```python
from build123d import *

# Parameters (mm, degrees)
SKETCH1_W           = 90
SKETCH1_H           = 20
BOSS_EXTRUDE1_DEPTH = 1
SKETCH2_R           = 2
CUT_EXTRUDE1_DEPTH  = 2
FILLET1_R           = 3
SKETCH3_W           = 74
SKETCH3_H           = 5.275339083
BOSS_EXTRUDE2_DEPTH = 8
SKETCH4_W           = 16
SKETCH4_H           = 3
BOSS_EXTRUDE3_DEPTH = 4
SKETCH5_W           = 4
SKETCH5_H           = 1.5
BOSS_EXTRUDE4_DEPTH = 10
SKETCH6_W           = 24
SKETCH6_H           = 11
BOSS_EXTRUDE5_DEPTH = 10
CUT_EXTRUDE2_DEPTH  = 12


with BuildPart() as part:
    # Sketch1 → Boss-Extrude1 (new body)
    with BuildSketch(Plane(origin=(0, 0, 0), x_dir=(1, 0, 0), z_dir=(0, 1, 0))):
        with Locations((45, 10)):
            Rectangle(SKETCH1_W, SKETCH1_H)
    extrude(amount=BOSS_EXTRUDE1_DEPTH)

    # Sketch2 → Cut-Extrude1 (cut, through all)
    with BuildSketch(Plane(origin=(0, 1, 0), x_dir=(1, 0, 0), z_dir=(0, 1, 0))):
        with Locations((3, 17)):
            Circle(SKETCH2_R)
        with Locations((87, 17)):
            Circle(SKETCH2_R)
        with Locations((87, 3)):
            Circle(SKETCH2_R)
        with Locations((3, 3)):
            Circle(SKETCH2_R)
    extrude(amount=-CUT_EXTRUDE1_DEPTH, mode=Mode.SUBTRACT)

    # Fillet1
    fillet1_edges = [part.edges().sort_by_distance(p)[0] for p in [
        (0, 0.5, -20),
        (90, 0.5, -20),
        (90, 0.5, 0),
        (0, 0.5, 0),
    ]]
    fillet(fillet1_edges, radius=FILLET1_R)

    # Sketch3 → Boss-Extrude2 (add)
    with BuildSketch(Plane(origin=(0, 1, 0), x_dir=(1, 0, 0), z_dir=(0, 1, 0))):
        with Locations((45, 15.362330459)):
            Rectangle(SKETCH3_W, SKETCH3_H)
    extrude(amount=BOSS_EXTRUDE2_DEPTH)

    # Sketch4 → Boss-Extrude3 (add)
    with BuildSketch(Plane(origin=(0, 1, 0), x_dir=(1, 0, 0), z_dir=(0, 1, 0))):
        with Locations((16, 2.5)):
            Rectangle(SKETCH4_W, SKETCH4_H)
    extrude(amount=BOSS_EXTRUDE3_DEPTH)

    # Sketch5 → Boss-Extrude4 (add)
    with BuildSketch(Plane(origin=(0, 9, 0), x_dir=(1, 0, 0), z_dir=(0, 1, 0))):
        with Locations((25, 15.362330459)):
            Rectangle(SKETCH5_W, SKETCH5_H)
    extrude(amount=BOSS_EXTRUDE4_DEPTH)

    # Sketch6 → Boss-Extrude5 (add)
    with BuildSketch(Plane(origin=(0, 19, 0), x_dir=(1, 0, 0), z_dir=(0, 1, 0))):
        with Locations((25, 15.362330459)):
            Rectangle(SKETCH6_W, SKETCH6_H)
    extrude(amount=BOSS_EXTRUDE5_DEPTH)

    # Sketch7 → Cut-Extrude2 (cut, through all)
    with BuildSketch(Plane.XY.offset(-9.862330459)):
        Polygon((37, 29), (25, 25.5), (13, 29), align=None)
    extrude(amount=-CUT_EXTRUDE2_DEPTH, mode=Mode.SUBTRACT)


solid = part.part
```
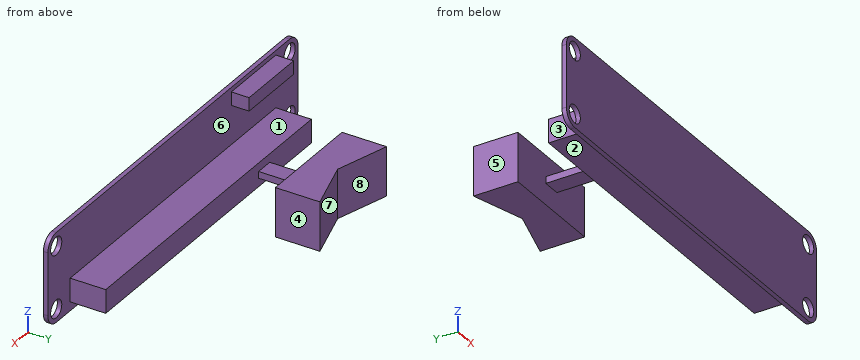
Part model, mm, in its own coordinate system. Face numbers are marked on the shaded views. A direction names the side the tool comes from. Round coordinates to 2 decimals unless told otherwise and drop trailing zeros. Order: outer loops, then holes, each group sorted by start corner. A loop starts at its lowest first (then second) coordinate and runs counter-clockwise, first axis right, second up. Notation, with made-up numbers: M 62.25,-1 L 101.25,-1 A21 cw 101.25,20 Z; hole C -29,30 d11. An arc over 180 degrees is marked long. Put each result on its own line as item: value. Start each with the question number.
1. Two-plate mould, pull along X, no slides. Class the marked faces 5, 6, 7 and 8: +X half, -X half, draft (parallel to the pull), parting line (faces both ways), or undercut.
2. Drop flat-ended pins along their axis: pin 1 (2 mm diameter, centred on x = 24, y = 12, fed in from +Z); pin 2 (1.6 mm diameter, centred on y = 12, z = -15, fed in from +X); pin 3 (4.5 mm diameter, centred on x = 19, y = 3, fed in from -Z). Give the stop position or say it passes through.
3. Tool access for the marked faces 1, 2, 3 and 4: list every direction of +Z, -Z, +X, -X, +Y, -Y with a clear straight run to the whole face (end or side of a thin tool).
4. Slice it at C-C on x = 29.5. List the corners of the cut face in (y, z).
5. Slice it at A-A on y = 2.75. List the corners of the cut face in (x, z).
6. Slice it at B-B on x = 18. List the corners of the cut face in (y, z).
7. Slice it at D-D on z = -6.25. List the corners of the cut face in (x, y).
8. Drill centre lines: probe 1 along Z at (x, y) = (87, 0.45); probe 2 along X at (y, z) = (0.85, -17); probe 3 along Y at (x, z) = (85, -12.5). Where is each one in solid material? Low to high. Write a range as [from, to].
Findings:
1. face 5: -X half
1. face 6: draft
1. face 7: undercut
1. face 8: undercut
2. pin 1: z = -14.61
2. pin 2: x = 27
2. pin 3: z = -20
3. face 1: +X, -X
3. face 2: -Z, +X, -X
3. face 3: +Z, -Z, -X, +Y
3. face 4: +Z, -Z, +X, +Y
4. outline: M 0,-20 L 1,-20 L 1,-18 L 9,-18 L 9,-12.72 L 1,-12.72 L 1,0 L 0,0 Z; M 19,-20.86 L 26.81,-20.86 L 26.81,-9.86 L 19,-9.86 Z
5. outline: M 8,-18 L 82,-18 L 82,-12.72 L 8,-12.72 Z; M 8,-4 L 24,-4 L 24,-1 L 8,-1 Z
6. outline: M 0,-20 L 1,-20 L 1,-18 L 9,-18 L 9,-12.72 L 1,-12.72 L 1,-4 L 5,-4 L 5,-1 L 1,-1 L 1,0 L 0,0 Z; M 19,-20.86 L 27.54,-20.86 L 27.54,-9.86 L 19,-9.86 Z
7. outline: M 0,0 L 90,0 L 90,1 L 0,1 Z
8. probe 1: [-20, -19], [-15, -5], [-1, 0]
8. probe 2: [0, 1], [5, 85], [89, 90]
8. probe 3: [0, 1]
